The listing builds one solid part. Answer for the finished solid, in the listing's coordinates (mm). Face numbers are marked on the shaded views. A direction names the side the tool comes from. Give positions to 0.01 mm unless a question says otherwise; leave off trailing zeros. Order: outer loops, then holes, each group sorted by start corner. A loop starts at its lowest first (then second) coordinate and runs counter-clockwise, first axis right, second up. Notation, with made-up numbers: (-25.5, -8.75) - (-0.5, -8.75) arc R13 ccw to (-0.5, 6.25) - close; hole circle Ø7 at (-34.75, 53.5). An arc over 180 degrees is marked (long way). Write each question's results on one line, items separated by ' | '. Start each with the question number.
1. Flat-ended cylindrical pins translate along their axes: pin 1 (12 mm diameter, centred on y = -13.5, z = -6, fed in from -X); pin 2 (5 mm diameter, centred on y = -17, z = -30, fed in from -X); pin 3 (12 mm diameter, centred on x = -5.5, y = -23, fed in from -Z); pin 4 (12 mm diameter, centred on x = -12, z = -23, fed in from -Y). Find the tip coordinate at first contact, or state that the pin passes through.
2. Section D-D (z = 0) is taken. Give the vertices of the cut face in (x, y).
3. Section B-B (z = -30) is taken. Give the vertices of the cut face in (x, y), and give its area (3 significant figures).
4. Find the intervals of material crossed by L1, parallel to Y at x = 30, z = 0; L2, parallel to X at y = 34, z = 10; L3, parallel to Z at x = -15.5, y = 11.5, in increasing order.
5. Section A-A (y = 0) is taken. Give the vertices of the cut face in (x, z).
6. Determine the mould class of the marked faces 1, 2 and 3 for opening direction Z: released by +Z, released by -Z, zero draft, split by the parting line, or undercut.
7. Section C-C (x = 2) is taken. Give the vertices of the cut face in (y, z), and give its area (3 significant figures).
8. Which of the six approach directions +Z, -Z, +X, -X, +Y, -Y give full straight-line access (tool end or side, diameter ignored) to the marked faces 4, 5 and 6?
from build123d import *

# Parameters (mm, degrees)
F3_D     = 6.8
F3_DEPTH = 48.75
F3_TIP   = 2.0429261047


with BuildPart() as f1:
    # F0 (on Front) → F1 (revolve)
    with BuildSketch(Plane.XZ):
        Polygon((4, 37.5), (0, 37.5), (0, 25), (-20, 25), (-20, 16), (45.9, 16), (45.9, 13), (50, 13), (50, 25), (4, 25), align=None)
    revolve(axis=Axis((40.2727089822, 0, 0), (1, 0, 0)))

    # F3
    with Locations(Plane.YZ.offset(4)):
        with Locations((0, -30), (-28.5316954889, -9.2705098312), (17.6335575688, 24.2705098312), (-17.6335575688, 24.2705098312), (28.5316954889, -9.2705098312)):
            Hole(F3_D / 2, depth=F3_DEPTH)
            with Locations((0, 0, -(F3_DEPTH + F3_TIP / 2))):  # 118° drill point
                Cone(0, F3_D / 2, F3_TIP, mode=Mode.SUBTRACT)


solid = f1.part
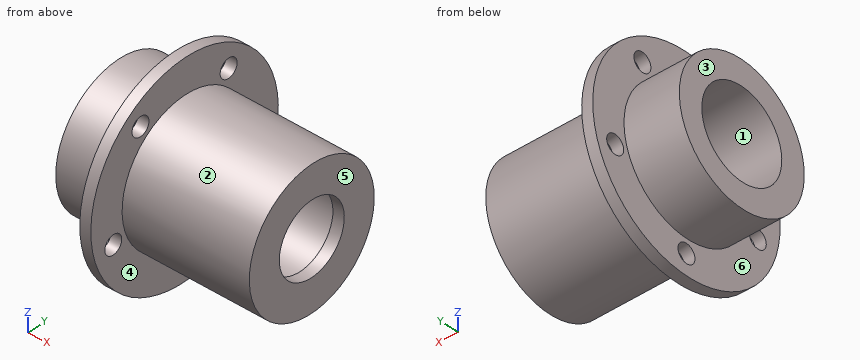
Reported:
1) pin 1: x = -20 | pin 2: x = 0 | pin 3: z = -31.33 | pin 4: y = -18.33
2) outline: (-20, -25) - (0, -25) - (0, -37.5) - (4, -37.5) - (4, -25) - (50, -25) - (50, -13) - (45.9, -13) - (45.9, -16) - (-20, -16) - close; (-20, 16) - (45.9, 16) - (45.9, 13) - (50, 13) - (50, 25) - (4, 25) - (4, 37.5) - (0, 37.5) - (0, 25) - (-20, 25) - close
3) outline: (0, -22.5) - (4, -22.5) - (4, -3.4) - (0, -3.4) - close; (0, 3.4) - (4, 3.4) - (4, 22.5) - (0, 22.5) - close | area: 153 mm²
4) L1: -25 to -16, 16 to 25 | L2: 0 to 4 | L3: -22.2 to -11.12, 11.12 to 22.2
5) outline: (-20, -25) - (0, -25) - (0, -26.6) - (4, -26.6) - (4, -25) - (50, -25) - (50, -13) - (45.9, -13) - (45.9, -16) - (-20, -16) - close; (-20, 16) - (45.9, 16) - (45.9, 13) - (50, 13) - (50, 25) - (4, 25) - (4, 37.5) - (0, 37.5) - (0, 25) - (-20, 25) - close; (0, -37.5) - (4, -37.5) - (4, -33.4) - (0, -33.4) - close
6) face 1: undercut | face 2: split by the parting line | face 3: zero draft
7) outline: circle Ø75 at (0, 0); hole circle Ø6.8 at (-28.53, -9.27); hole circle Ø6.8 at (-17.63, 24.27); hole circle Ø32 at (0, 0); hole circle Ø6.8 at (0, -30); hole circle Ø6.8 at (17.63, 24.27); hole circle Ø6.8 at (28.53, -9.27) | area: 3,430 mm²
8) face 4: +X | face 5: +Z, -Z, +X, +Y, -Y | face 6: -X
